from build123d import *

# Parameters (mm, degrees)
BOSS_EXTRUDE1_DEPTH     = 2.54
CUT_EXTRUDE1_DEPTH      = 1
CUT_EXTRUDE1_DEPTH_BACK = 3.54
CUT_EXTRUDE2_DEPTH      = 7.62


with BuildPart() as part:
    # Sketch1 → Boss-Extrude1 (new body)
    with BuildSketch(Plane.XY):
        Polygon((-945.957227657, 86.137779906), (-945.969713578, 86.1172966), (-949.121092485, 86.403457059), (-949.65244679, 80.075727402), (-9.887238192, -5.25964904), (-6.723373364, -5.525326193), (0, -5.833733414), (152.4, -5.833733414), (152.4, 11.946266586), (139.7, 11.946266586), (139.7, 6.866266586), (136.525, 6.866266586), (136.525, 11.946266586), (95.25, 11.946266586), (95.25, 6.866266586), (92.075, 6.866266586), (92.075, 11.946266586), (79.375, 11.946266586), (79.375, 6.866266586), (76.2, 6.866266586), (76.2, 11.946266586), (69.85, 11.946266586), (25.4, 19.566266586), (19.05, 19.566266586), (19.05, 14.486266586), (15.875, 14.486266586), (15.875, 19.566266586), (3.175, 19.566266586), (3.175, 13.216266586), (0, 13.216266586), (0, 19.566266586), (-1.98607431, 19.566266586), (-4.597956143, 19.785592432), (-5.129310448, 13.457862776), (-8.293175277, 13.723539928), (-7.761820971, 20.051269584), (-944.89858306, 98.744842179), align=None)
    extrude(amount=BOSS_EXTRUDE1_DEPTH)

    # Sketch2 → Cut-Extrude1 (cut, two sides)
    with BuildSketch(Plane.XY.offset(2.54)) as cut_extrude1_sk:
        Polygon((-867.4716203, 85.879017088), (-866.940953695, 92.198557139), (-870.104818523, 92.464234292), (-870.635482595, 86.144724398), align=None)
        Polygon((-788.501617399, 79.246962625), (-787.970887585, 85.567255411), (-791.134752413, 85.832932563), (-791.665479694, 79.512669935), align=None)
        Polygon((-709.531614498, 72.614908162), (-709.000821475, 78.935953682), (-712.164686303, 79.201630835), (-712.695476794, 72.880615473), align=None)
        Polygon((-630.561611597, 65.9828537), (-630.030755365, 72.304651954), (-633.194620194, 72.570329107), (-633.725473893, 66.24856101), align=None)
        Polygon((-551.591608696, 59.350799237), (-551.060689256, 65.673350226), (-554.224554084, 65.939027378), (-554.755470992, 59.616506547), align=None)
        Polygon((-472.621605795, 52.718744774), (-472.090623146, 59.042048497), (-475.254487974, 59.30772565), (-475.785468091, 52.984452084), align=None)
        Polygon((-393.651602894, 46.086690311), (-393.120557036, 52.410746769), (-396.284421864, 52.676423921), (-396.81546519, 46.352397622), align=None)
        Polygon((-314.681599993, 39.454635849), (-314.150490926, 45.77944504), (-317.314355754, 46.045122193), (-317.845462289, 39.720343159), align=None)
        Polygon((-235.711597092, 32.822581386), (-235.180424816, 39.148143312), (-238.344289645, 39.413820465), (-238.875459388, 33.088288696), align=None)
        Polygon((-156.741594191, 26.190526923), (-156.210358707, 32.516841584), (-159.374223535, 32.782518736), (-159.905456487, 26.456234233), align=None)
        Polygon((-77.240292597, 25.885539855), (-80.404157425, 26.151217008), (-80.935453586, 19.824179771), (-77.77159129, 19.55847246), align=None)
    extrude(amount=CUT_EXTRUDE1_DEPTH, mode=Mode.SUBTRACT)
    extrude(cut_extrude1_sk.sketch, amount=-CUT_EXTRUDE1_DEPTH_BACK, mode=Mode.SUBTRACT)

    # Sketch3 → Cut-Extrude2 (cut)
    with BuildSketch(Plane.XY.offset(2.54)):
        Polygon((-434.187522505, 55.859236209), (-441.444486836, 50.074133547), (-431.803024179, 44.022577198), (-442.349656028, 39.171455119), (-433.014300591, 33.162402364), (-1000.074058288, -11.780320021), (-979.22273749, 133.880780984), align=None)
    extrude(amount=-CUT_EXTRUDE2_DEPTH, mode=Mode.SUBTRACT)


solid = part.part
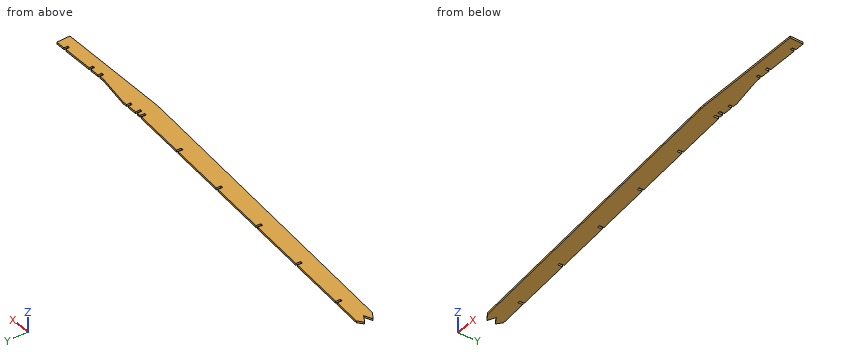
For this review, take the finished solid that the model builds, in its own axes (mm). Coordinates: 2 decimals unless noted, no trailing zeros. Loops run counter-clockwise (first coordinate to the right, second up) from the corner with the lowest first, then second, coordinate; pieces in that order, holes last. Notation, with made-up numbers: (-32.75, -8.75) - (19.25, -8.75) arc R22 ccw to (19.25, 15.25) - close; hole circle Ø6 at (77, 40). An arc over 180 degrees is marked (long way). Use a Markdown table: item, result. Add a question column.
Item 1: Insertion check: pin 1 Ø1.3 at (x, z) = (89, 1.5) entering from +Y; pin 2 Ø0.8 at (x, z) = (93, 1.5) entering from +Y; pin 3 Ø0.8 at (x, z) = (6.5, 1) entering from +Y. Each pin has a flat end and moves straight along its axis. Give the tip position at first contact, or say it passes through.
Item 2: For line 1 (Y direction, x = 110, z = 0.6); line 2 (Y direction, x = 24, z = 1.7); line 3 (X direction, y = 46, z = 1.3), list the stretches that pass through material, from the lowest coordinate up.
Item 3: We need section B-B (x = -371). Give the boundary of the cut face in (y, z).
Item 4: We need section A-A (x = -203.5). Give the boundary of the cut face in (y, z).
Results list:
| question | item | result |
|---|---|---|
| 1 | pin 1 | stops at y = 11.95 |
| 1 | pin 2 | stops at y = 6.87 |
| 1 | pin 3 | stops at y = 19.57 |
| 2 | line 1 | y = -5.83 to 11.95 |
| 2 | line 2 | y = -5.83 to 19.57 |
| 2 | line 3 | x = -434.95 to -317.32 |
| 3 | outline | (27.53, 0) - (50.55, 0) - (50.55, 2.54) - (27.53, 2.54) - close |
| 4 | outline | (12.32, 0) - (36.49, 0) - (36.49, 2.54) - (12.32, 2.54) - close |
